The drawing under review shows one solid part. Ordinate dimensions are in mm from its lowest x, y, z. Coordinates: 2 decimals unless noted, no trailing zeros. Loops run counter-clockwise (first coordinate to the right, second up) from the corner with the lowest first, then second, coordinate; pieces in that order, holes last. Notation, with made-up numbers: (17, 25) - (26, 25) arc R16 ccw to (26, 55) - close; hole circle Ø3 at (36, 7). An arc over 180 degrees is marked (long way). Answer as a JSON object with one key per item and string values. Group by question number.
Item 1: Clearance check with flat-ended pins moving along their axes: pin 1 (1.5 mm diameter, centred on x = 1, y = 8.5, fed in from +Z); pin 2 (1 mm diameter, centred on x = 2, z = 18, fed in from -Y); pin 3 (1 mm diameter, centred on x = 1, y = 6, fed in from +Z). State where each tip first meets the part, or that it passes through.
Item 2: We need section B-B (z = 19). Give the boundary of the cut face in (x, y).
Item 3: We need section A-A (z = 15). Give the boundary of the cut face in (x, y).
Item 4: Mouldability with a two-part tool opening along Z and no side actions: class the marked faces 1, 2, 3 and 4 as released by +Z, released by -Z, zero draft, split by the parting line, or undercut.
Item 5: To check wall thickness, follow line 1 (Y direction, x = 0.9, z = 15); line 2 (Y direction, x = 0.5, z = 6.75); line 3 (Y direction, x = 1.65, z = 23.5). State the ranges of each line that lie inside material, in increasing order.
Item 6: We need section C-C (y = 9). Give the boundary of the cut face in (x, z), then the cut area to 3 significant figures.
Item 7: We need section D-D (x = 0.7). State how many separate pieces and enclosed holes the cut face has.
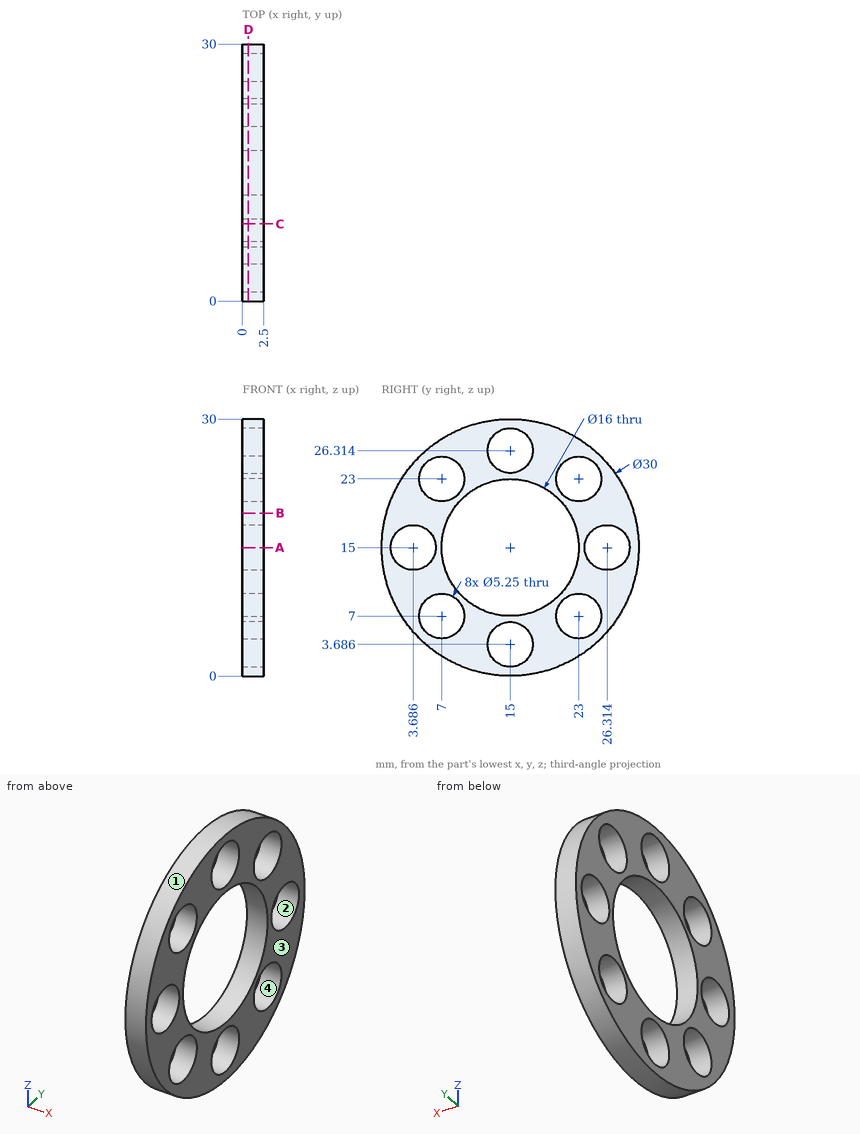
Check sheet entries:
{
 "1": {"pin 1": "stops at z = 28.85", "pin 2": "stops at y = 0.21", "pin 3": "stops at z = 27.36"},
 "2": {"outline": "(0, 0.54) - (2.5, 0.54) - (2.5, 8.07) - (0, 8.07) - close; (0, 21.93) - (2.5, 21.93) - (2.5, 29.46) - (0, 29.46) - close"},
 "3": {"outline": "(0, 0) - (2.5, 0) - (2.5, 1.06) - (0, 1.06) - close; (0, 6.31) - (2.5, 6.31) - (2.5, 7) - (0, 7) - close; (0, 23) - (2.5, 23) - (2.5, 23.69) - (0, 23.69) - close; (0, 28.94) - (2.5, 28.94) - (2.5, 30) - (0, 30) - close"},
 "4": {"face 1": "split by the parting line", "face 2": "undercut", "face 3": "zero draft", "face 4": "undercut"},
 "5": {"line 1": "y = 0 to 1.06, 6.31 to 7, 23 to 23.69, 28.94 to 30", "line 2": "y = 2.47 to 4.39, 9.61 to 20.39, 25.61 to 27.53", "line 3": "y = 2.64 to 4.42, 9.58 to 20.42, 25.58 to 27.36"},
 "6": {"outline": "(0, 1.25) - (2.5, 1.25) - (2.5, 5.3) - (0, 5.3) - close; (0, 8.7) - (2.5, 8.7) - (2.5, 9.71) - (0, 9.71) - close; (0, 20.29) - (2.5, 20.29) - (2.5, 21.3) - (0, 21.3) - close; (0, 24.7) - (2.5, 24.7) - (2.5, 28.75) - (0, 28.75) - close", "area": "25.3 mm2"},
 "7": {"separate pieces": "1", "enclosed holes": "9"}
}
